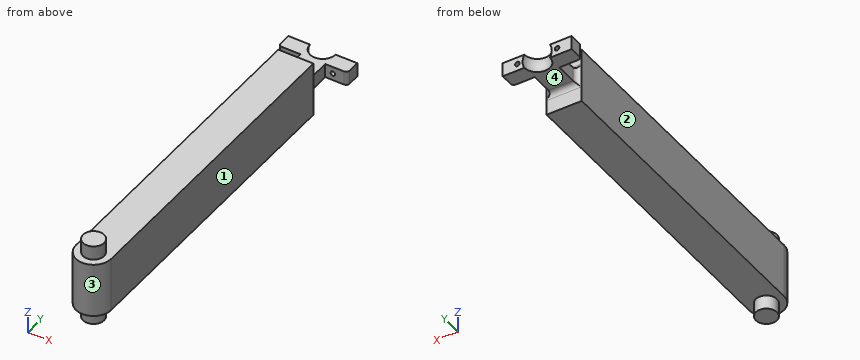
from build123d import *

# Parameters (mm, degrees)
EXTRUDE_1_DEPTH = 7.8
SKETCH_4_R      = 3
EXTRUDE_3_DEPTH = 4
SKETCH_5_W      = 7
SKETCH_5_H      = 4
EXTRUDE_4_DEPTH = 12
SKETCH_7_W      = 19.6
SKETCH_7_H      = 4.4
EXTRUDE_5_DEPTH = 2
FILLET_2_R      = 1
HOLE_WIZARD_1_D = 1.3
FILLET_3_R      = 1.5


with BuildPart() as part:
    # 草图1 → 凸台-拉伸1 (new, symmetric)
    with BuildSketch(Plane.XY):
        with BuildLine():
            Line((5, 0), (5, 90))
            Line((5, 90), (-5, 90))
            Line((-5, 90), (-5, 0))
            ThreePointArc((-5, 0), (0, -5), (5, 0))
        make_face()
    extrude(amount=EXTRUDE_1_DEPTH, both=True)

    # 草图4 → 凸台-拉伸3 (add)
    with BuildSketch(Plane.XY.offset(7.8)):
        Circle(SKETCH_4_R)
    extrude_3 = extrude(amount=EXTRUDE_3_DEPTH)

    # 草图5 → 凸台-拉伸4 (add)
    with BuildSketch(Plane(origin=(0, 102, 0), x_dir=(1, 0, 0), z_dir=(0, 1, 0))):
        Rectangle(SKETCH_5_W, SKETCH_5_H)
    extrude(amount=-EXTRUDE_4_DEPTH)

    # 草图7 → 凸台-拉伸5 (add, symmetric)
    with BuildSketch(Plane.XY):
        with Locations((0, 99.8)):
            Rectangle(SKETCH_7_W, SKETCH_7_H)
    extrude(amount=EXTRUDE_5_DEPTH, both=True)

    # 草图10 → 切除-旋转1 (revolve, cut)
    with BuildSketch(Plane.XY):
        with BuildLine():
            ThreePointArc((4.15, 102), (2.934493142, 104.934493142), (0, 106.15))
            Line((0, 106.15), (0, 102))
            Line((0, 102), (0, 97.85))
            ThreePointArc((0, 97.85), (2.934493142, 99.065506858), (4.15, 102))
        make_face()
    revolve(axis=Axis((0, 106.15, 0), (0, -1, 0)), mode=Mode.SUBTRACT)

    # 镜向2: 凸台-拉伸3 across plane
    add(extrude_3.mirror(Plane.XY))

    # 圆角2
    fillet_2_edges = [part.edges().sort_by_distance(p)[0] for p in [
        (-9.8, 97.6, 0),
        (9.8, 97.6, 0),
    ]]
    fillet(fillet_2_edges, radius=FILLET_2_R)

    # 孔1 (through all)
    with Locations(Plane(origin=(0, 97.6, 0), x_dir=(-1, 0, 0), z_dir=(0, -1, 0))):
        with Locations((5.65, 0), (-5.65, 0)):
            Hole(HOLE_WIZARD_1_D / 2)

    # 圆角3
    fillet_3_edges = [part.edges().sort_by_distance(p)[0] for p in [
        (0, 90, -2),
        (-3.5, 90, 0),
        (0, 90, 2),
        (3.5, 90, 0),
    ]]
    fillet(fillet_3_edges, radius=FILLET_3_R - 0.0001)  # a hair under: the kernel refuses the full size


solid = part.part
The listing builds one solid part. Answer for the finished solid, in the listing's coordinates (mm). Face numbers are marked on the shaded views. A direction names the side the tool comes from. Round coordinates to 2 decimals unless told otherwise and drop trailing zeros. Write each loop counter-clockwise with the first axis right and the second up, starting at its lowest first coordinate (ties: lowest second). Pieces come first, ordered by that corner, then holes. Notation, with made-up numbers: M -4.75,-25 L 18.25,-25 A11 ccw 18.25,-11 Z; hole C -8.75,72.5 d9. An arc over 180 degrees is marked long. Write each question's results on one line, items separated by ' | '. Start each with the question number.
Item 1: Find section D-D on z = 10. Write down the section's boundary in (x, y).
Item 2: Given pin 1 Ø8 at (y, z) = (19, 0) entering from +X; pin 2 Ø11.5 at (x, y) = (4, 96.5) entering from +Z; pin 3 Ø5.5 at (x, y) = (-3.5, 98.5) entering from -Z, each flat-ended and moving along its own axis, determine where each tip first touches the part or whether it passes through.
Item 3: Straight lines are drawn through the part: probe 1 along Z at (x, y) = (5.65, 99.6); probe 2 along Y at (x, z) = (-4, 3.25); probe 3 along Z at (x, y) = (0.75, 4.5). For each, find the intervals that lie inside material, in ascending order.
Item 4: Which of the six approach directions +Z, -Z, +X, -X, +Y, -Y give full straight-line access (tool end or side, diameter ignored) to the marked faces 1, 2, 3 and 4?
Item 5: Find section C-C on x = 0. Write down the section's boundary in (y, z), and give its area (3 significant figures).
Item 6: Find section A-A on z = 4.5. Write down the section's boundary in (x, y).
Item 7: Find section B-B on y = 17. Write down the section's boundary in (x, z).
Answer block:
1) outline: C 0,0 d6
2) pin 1: stops at x = 5 | pin 2: stops at z = 2.2 | pin 3: stops at z = -2
3) probe 1: z = -2 to -0.65, 0.65 to 2 | probe 2: y = -3 to 90.02 | probe 3: z = -7.8 to 7.8
4) face 1: +Z, -Z, +X, -Y | face 2: +Z, -Z, -X, -Y | face 3: +Z, -Z, -Y | face 4: -Z, +X, -X, +Y
5) outline: M -5,-7.8 L -3,-7.8 L -3,-11.8 L 3,-11.8 L 3,-7.8 L 90,-7.8 L 90,-3.5 A1.5 cw 91.5,-2 L 98.36,-2 A4.15 cw 98.36,2 L 91.5,2 A1.5 cw 90,3.5 L 90,7.8 L 3,7.8 L 3,11.8 L -3,11.8 L -3,7.8 L -5,7.8 Z | area: 1,560 mm²
6) outline: M -5,0 A5 ccw 5,0 L 5,90 L -5,90 Z
7) outline: M -5,-7.8 L 5,-7.8 L 5,7.8 L -5,7.8 Z
